Part model, mm, in its own coordinate system. Coordinates: 2 decimals unless noted, no trailing zeros. Write each loop counter-clockwise with the first axis right and the second up, starting at its lowest first coordinate (ties: lowest second). Pieces come first, ordered by that corner, then holes. Notation, with made-up numbers: (-9, 82) - (10, 82) arc R16 ccw to (10, 99) - close; hole circle Ø8 at (-1.5, 2). An arc over 180 degrees is marked (long way). Write each question's results on one line, items separated by ' | '.
from build123d import *

# Parameters (mm, degrees)
F0_W     = 550
F0_H     = 270
F1_DEPTH = 13
F2_R     = 2.5
F3_DEPTH = 25
F4_R     = 5
F5_R     = 20


with BuildPart() as f1:
    # F0 (on Top) → F1 (new body)
    with BuildSketch(Plane.XY):
        with Locations((275, -135)):
            Rectangle(F0_W, F0_H)
    extrude(amount=-F1_DEPTH)

    # F2 (on face) → F3 (cut)
    with BuildSketch(Plane.XY):
        with BuildLine():
            ThreePointArc((102.8172889589, -52.4701250099), (119.1726628165, -90.0990620723), (143.6244940218, -123.0466433063))
            ThreePointArc((143.6244940218, -123.0466433063), (145.375436454, -115.11981647), (145.9631920321, -107.023216784))
            ThreePointArc((145.9631920321, -107.023216784), (133.8730301026, -72.2467564476), (102.8172889589, -52.4701250099))
        make_face()
        with BuildLine():
            ThreePointArc((46.4524007703, -71.5977994519), (67.6630708031, -119.8818075906), (98.9269281749, -162.353082441))
            ThreePointArc((98.9269281749, -162.353082441), (126.0574308053, -149.8675419291), (142.9268949098, -125.2225814773))
            ThreePointArc((142.9268949098, -125.2225814773), (117.4412479589, -91.100162762), (100.5834584289, -51.9891337337))
            ThreePointArc((100.5834584289, -51.9891337337), (70.8084957225, -54.3138897804), (46.4524007703, -71.5977994519))
        make_face()
        with BuildLine():
            ThreePointArc((36.6062109858, -22.9924196081), (40.2678425285, -47.5506492992), (46.4524007703, -71.5977994519))
            ThreePointArc((46.4524007703, -71.5977994519), (70.8084957225, -54.3138897804), (100.5834584289, -51.9891337337))
            ThreePointArc((100.5834584289, -51.9891337337), (96.3763447636, -34.89397928), (93.8406279725, -17.4723188671))
            Line((93.8406279725, -17.4723188671), (36.6062109858, -22.9924196081))
        make_face()
        with BuildLine():
            ThreePointArc((26.1547087534, -24.0004380043), (30.8880481953, -53.9384370008), (39.2095922874, -83.0835942334))
            ThreePointArc((39.2095922874, -83.0835942334), (42.4819606163, -77.1205988593), (46.4524007703, -71.5977994519))
            ThreePointArc((46.4524007703, -71.5977994519), (40.2678425285, -47.5506492992), (36.6062109858, -22.9924196081))
            Line((36.6062109858, -22.9924196081), (26.1547087534, -24.0004380043))
        make_face()
        with BuildLine():
            ThreePointArc((39.2095922874, -83.0835942334), (58.5731428007, -125.1375862115), (85.359218008, -162.8998889056))
            ThreePointArc((85.359218008, -162.8998889056), (92.159689712, -163.0387878421), (98.9269281749, -162.353082441))
            ThreePointArc((98.9269281749, -162.353082441), (67.6630708031, -119.8818075906), (46.4524007703, -71.5977994519))
            ThreePointArc((46.4524007703, -71.5977994519), (42.4819606163, -77.1205988593), (39.2095922874, -83.0835942334))
        make_face()
        with BuildLine():
            ThreePointArc((39.2095922874, -83.0835942334), (41.3696850637, -135.0845918815), (85.359218008, -162.8998889056))
            ThreePointArc((85.359218008, -162.8998889056), (58.5731428007, -125.1375862115), (39.2095922874, -83.0835942334))
        make_face()
        with BuildLine():
            ThreePointArc((98.9269281749, -162.353082441), (129.5126452175, -190.2463655327), (164.4445024089, -212.4564236553))
            Line((164.4445024089, -212.4564236553), (190.9870540226, -161.4491403142))
            ThreePointArc((190.9870540226, -161.4491403142), (165.4491613095, -145.3362093293), (142.9268949098, -125.2225814773))
            ThreePointArc((142.9268949098, -125.2225814773), (126.0574308053, -149.8675419291), (98.9269281749, -162.353082441))
        make_face()
        with BuildLine():
            ThreePointArc((85.359218008, -162.8998889056), (119.6639725539, -195.884452107), (159.5976016794, -221.7707971349))
            Line((159.5976016794, -221.7707971349), (164.4445024089, -212.4564236553))
            ThreePointArc((164.4445024089, -212.4564236553), (129.5126452175, -190.2463655327), (98.9269281749, -162.353082441))
            ThreePointArc((98.9269281749, -162.353082441), (92.159689712, -163.0387878421), (85.359218008, -162.8998889056))
        make_face()
        with BuildLine():
            ThreePointArc((142.9268949098, -125.2225814773), (165.4491613095, -145.3362093293), (190.9870540226, -161.4491403142))
            Line((190.9870540226, -161.4491403142), (191.9102732092, -159.6749739371))
            ThreePointArc((191.9102732092, -159.6749739371), (166.2146946142, -143.4076613439), (143.6244940218, -123.0466433063))
            ThreePointArc((143.6244940218, -123.0466433063), (143.2867819227, -124.1381669965), (142.9268949098, -125.2225814773))
        make_face()
        with BuildLine():
            Line((190.9870540226, -161.4491403142), (164.4445024089, -212.4564236553))
            ThreePointArc((164.4445024089, -212.4564236553), (312.3186805101, -236.5746522453), (445.5878496959, -168.1072144083))
            ThreePointArc((445.5878496959, -168.1072144083), (417.7995521532, -156.6837386519), (396.3969974723, -135.5978207964))
            ThreePointArc((396.3969974723, -135.5978207964), (297.7258554679, -180.5755672655), (190.9870540226, -161.4491403142))
        make_face()
        with BuildLine():
            ThreePointArc((396.3969974723, -135.5978207964), (417.7995521532, -156.6837386519), (445.5878496959, -168.1072144083))
            ThreePointArc((445.5878496959, -168.1072144083), (489.778644371, -105.9735057557), (512.2017629268, -33.0994511193))
            ThreePointArc((512.2017629268, -33.0994511193), (486.2288437534, -17.9967113583), (456.4729635167, -13.8406471114))
            ThreePointArc((456.4729635167, -13.8406471114), (438.2138341358, -80.5310148123), (396.3969974723, -135.5978207964))
        make_face()
        with BuildLine():
            ThreePointArc((395.2793152892, -133.9137271289), (395.8326968589, -134.7593972826), (396.3969974723, -135.5978207964))
            ThreePointArc((396.3969974723, -135.5978207964), (438.2138341358, -80.5310148123), (456.4729635167, -13.8406471114))
            ThreePointArc((456.4729635167, -13.8406471114), (391.3304963156, -56.2714595868), (395.2793152892, -133.9137271289))
        make_face()
        with BuildLine():
            ThreePointArc((445.5878496959, -168.1072144083), (452.1119253863, -169.1179747106), (458.6981361528, -169.5729777234))
            ThreePointArc((458.6981361528, -169.5729777234), (515.1450884683, -147.5010120731), (538.711061865, -91.6612861494))
            ThreePointArc((538.711061865, -91.6612861494), (531.7751165183, -59.5200686387), (512.2017629268, -33.0994511193))
            ThreePointArc((512.2017629268, -33.0994511193), (489.778644371, -105.9735057557), (445.5878496959, -168.1072144083))
        make_face()
        with BuildLine():
            ThreePointArc((17.5, -255), (13.232233047, -253.232233047), (15, -257.5))
            ThreePointArc((15, -257.5), (16.767766953, -256.767766953), (17.5, -255))
        make_face()
        with Locations((15, -15)):
            Circle(F2_R)
        with BuildLine():
            ThreePointArc((537.5, -15), (536.767766953, -13.232233047), (535, -12.5))
            ThreePointArc((535, -12.5), (533.232233047, -16.767766953), (537.5, -15))
        make_face()
        with Locations((535, -255)):
            Circle(F2_R)
        with BuildLine():
            ThreePointArc((100.5834584289, -51.9891337337), (117.4412479589, -91.100162762), (142.9268949098, -125.2225814773))
            ThreePointArc((142.9268949098, -125.2225814773), (143.2867819227, -124.1381669965), (143.6244940218, -123.0466433063))
            ThreePointArc((143.6244940218, -123.0466433063), (119.1726628165, -90.0990620723), (102.8172889589, -52.4701250099))
            ThreePointArc((102.8172889589, -52.4701250099), (101.702824577, -52.2182469254), (100.5834584289, -51.9891337337))
        make_face()
        with BuildLine():
            ThreePointArc((93.8406279725, -17.4723188671), (96.3763447636, -34.89397928), (100.5834584289, -51.9891337337))
            ThreePointArc((100.5834584289, -51.9891337337), (101.702824577, -52.2182469254), (102.8172889589, -52.4701250099))
            ThreePointArc((102.8172889589, -52.4701250099), (98.4454239564, -35.0497029669), (95.8313903025, -17.2803153631))
            Line((95.8313903025, -17.2803153631), (93.8406279725, -17.4723188671))
        make_face()
    extrude(amount=-F3_DEPTH, mode=Mode.SUBTRACT)

    # F4
    f4_edges = [f1.edges().sort_by_distance(p)[0] for p in [
        (102.817289, -52.470125, -6.5),
        (143.624494, -123.046643, -6.5),
        (39.209592, -83.083594, -6.5),
        (85.359218, -162.899889, -6.5),
        (396.396997, -135.597821, -6.5),
    ]]
    fillet(f4_edges, radius=F4_R)

    # F5
    f5_edges = [f1.edges().sort_by_distance(p)[0] for p in [
        (445.58785, -168.107214, -6.5),
    ]]
    fillet(f5_edges, radius=F5_R)


solid = f1.part
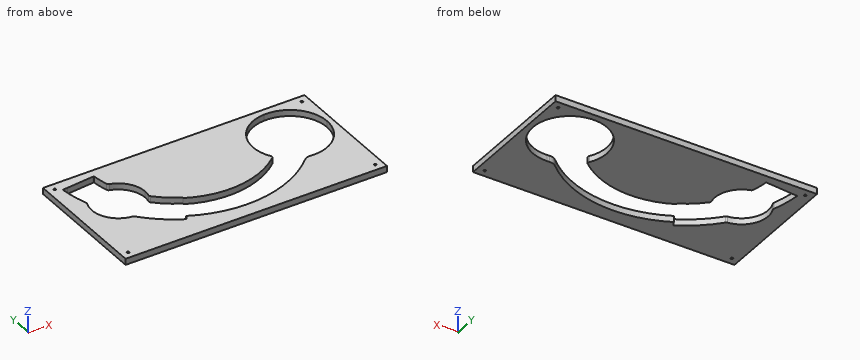
(1) Saw through at D-D on y = -39.5. Write the cut outline in (x, z).
Return value:
outline: (0, -13) - (28.14, -13) - (28.14, 0) - (0, 0) - close; (99.39, -13) - (402.86, -13) - (402.86, 0) - (99.39, 0) - close; (518.68, -13) - (550, -13) - (550, 0) - (518.68, 0) - close
(2) Saw through at A-A on y = -147. Write the cut outline in (x, z).
Return value:
outline: (0, -13) - (50.6, -13) - (50.6, 0) - (0, 0) - close; (171.12, -13) - (382.31, -13) - (382.31, 0) - (171.12, 0) - close; (515.65, -13) - (550, -13) - (550, 0) - (515.65, 0) - close
(3) Saw through at B-B on y = -197. Write the cut outline in (x, z), then the cut area to 3 significant figures.
Return value:
outline: (0, -13) - (121.08, -13) - (121.08, 0) - (0, 0) - close; (411.2, -13) - (550, -13) - (550, 0) - (411.2, 0) - close | area: 3,380 mm^2
(4) Wall check: line 1 (X direction, y = -255, z = -2.5); line 2 (Y direction, x = 458, z = -0.75); line 3 (Y direction, x = 270, z = -7). Give the ranges that are in metal, low to high. Write a range as from..to.
Return value:
line 1: x = 0..12.5, 17.5..532.5, 537.5..550 | line 2: y = -270..-169.55, -13.77..0 | line 3: y = -270..-239.45, -181.93..0
(5) Flat gauge pin, fed straight in: P1, Ø5, axis at y = -66.5, z = -3, coming from the -X side. Where does the tip first touch, or does it go through?
Return value:
P1: stops at x = 0
(6) Saw through at C-C on x = 343. Write the cut outline in (y, z).
Return value:
outline: (-270, -13) - (-229.64, -13) - (-229.64, 0) - (-270, 0) - close; (-168.82, -13) - (0, -13) - (0, 0) - (-168.82, 0) - close
